The drawing under review shows one solid part. Ordinate dimensions are in mm from its lowest x, y, z. A direction names the side the tool comes from. Round coordinates to 2 decimals unless told otherwise and drop trailing zeros. Order: outer loops, then holes, each group sorted by start corner. A loop starts at its lowest first (then second) coordinate and runs counter-clockwise, first axis right, second up. Notation, with made-up numbers: (44, 34) - (53, 34) arc R28 ccw to (53, 73) - close; hole circle Ø4 at (-4, 26). An arc over 180 degrees is marked (long way). Answer as a JSON object with one key per item and string values. Group by question number.
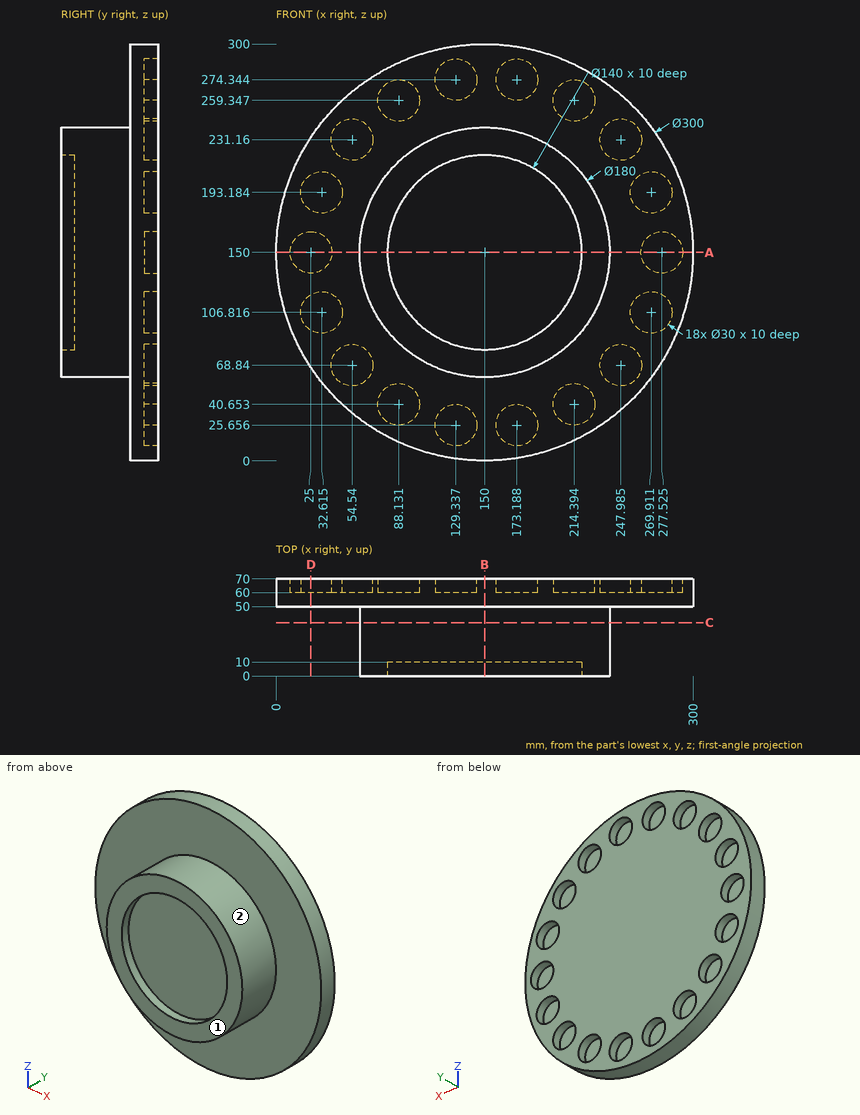
1. Take a section at B-B, the plane x = 150. Give the boundary of the cut face in (y, z).
2. Tool access review of the marked faces 1 and 2: name each direction out of +Z, -Z, +X, -X, +Y, -Y from which nothing blocks a thin tool from reaching the whole face with its end or side.
3. Clearance check with flat-ended pins moving along their axes: P1, Ø3, axis at y = 56, z = 32.5, coming from the +X side; P2, Ø2, axis at x = 105, y = 33.5, coming from the +Z side; P3, Ø8, axis at x = 144.5, z = 141.5, coming from the -Y side. State where each tip first meets the part, or that it passes through.
4. To check wall thickness, follow line 1 (X direction, y = 64, z = 150) (1 decimal); line 2 (X direction, y = 66.5, z = 261) (1 decimal); line 3 (Y direction, x = 136.5, z = 59.5). State the ranges of each line that lie inside material, in increasing order. Write a range as from..to.
5. Take a section at D-D, the plane x = 25. Give the boundary of the cut face in (y, z) (1 decimal).
6. Take a section at A-A, the plane z = 150. Give the boundary of the cut face in (x, y) (1 decimal), then the cut area to 3 significant figures.
7. Take a section at C-C, the plane y = 38.5. Give the boundary of the cut face in (x, z).
Response values:
{
 "1": {"outline": "(0, 60) - (50, 60) - (50, 0) - (70, 0) - (70, 300) - (50, 300) - (50, 240) - (0, 240) - (0, 220) - (10, 220) - (10, 80) - (0, 80) - close"},
 "2": {"face 1": "+Z, -Z, +X, -X, -Y", "face 2": "-Y"},
 "3": {"P1": "x = 245.1", "P2": "z = 228.51", "P3": "y = 10"},
 "4": {"line 1": "0..10, 40..262.5, 292.5..300", "line 2": "49.1..73.2, 103..122.5, 136.2..166.3, 180..199.5, 229.3..250.9", "line 3": "50..70"},
 "5": {"outline": "(50, 67.1) - (70, 67.1) - (70, 93.9) - (60, 93.9) - (60, 119.7) - (70, 119.7) - (70, 135) - (60, 135) - (60, 165) - (70, 165) - (70, 180.3) - (60, 180.3) - (60, 206.1) - (70, 206.1) - (70, 232.9) - (50, 232.9) - close"},
 "6": {"outline": "(0, 50) - (60, 50) - (60, 0) - (80, 0) - (80, 10) - (220, 10) - (220, 0) - (240, 0) - (240, 50) - (300, 50) - (300, 70) - (292.5, 70) - (292.5, 60) - (262.5, 60) - (262.5, 70) - (40, 70) - (40, 60) - (10, 60) - (10, 70) - (0, 70) - close", "area": "13,000 mm2"},
 "7": {"outline": "circle Ø180 at (150, 150)"}
}
